from build123d import *

# Parameters (mm, degrees)
CROQUIS1_W              = 3
CROQUIS1_H              = 12.3
SALIENTE_EXTRUIR1_DEPTH = 3


with BuildPart() as part:
    # Croquis1 → Saliente-Extruir1 (new body)
    with BuildSketch(Plane.XY):
        Polygon((307.259692282, 25.949980259), (346.230835452, 48.449980259), (346.230835452, 93.449980259), (307.259692282, 115.949980259), (268.288549111, 93.449980259), (268.288549111, 48.449980259), align=None)
        with Locations((307.259692282, 70.949980259)):
            Rectangle(CROQUIS1_W, CROQUIS1_H, mode=Mode.SUBTRACT)
        with Locations((332.809217745, 70.949980259)):
            Rectangle(CROQUIS1_W, CROQUIS1_H, mode=Mode.SUBTRACT)
        with Locations((281.710166819, 70.949980259)):
            Rectangle(CROQUIS1_W, CROQUIS1_H, mode=Mode.SUBTRACT)
        Polygon((313.95839878, 94.852480259), (324.610511247, 88.702480259), (326.110511247, 91.30055647), (315.45839878, 97.45055647), align=None, mode=Mode.SUBTRACT)
        Polygon((289.908873317, 88.702480259), (288.408873317, 91.30055647), (299.060985783, 97.45055647), (300.560985783, 94.852480259), align=None, mode=Mode.SUBTRACT)
        Polygon((300.560985783, 47.047480259), (289.908873317, 53.197480259), (288.408873317, 50.599404048), (299.060985783, 44.449404048), align=None, mode=Mode.SUBTRACT)
        Polygon((324.610511247, 53.197480259), (326.110511247, 50.599404048), (315.45839878, 44.449404048), (313.95839878, 47.047480259), align=None, mode=Mode.SUBTRACT)
    extrude(amount=SALIENTE_EXTRUIR1_DEPTH)


solid = part.part
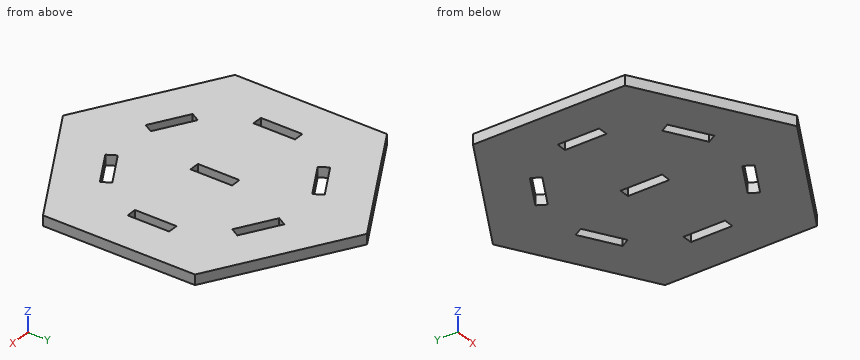
Work out the finished part from the listing and answer in its coordinate system (mm). Round coordinates to 2 decimals unless told otherwise and drop trailing zeros. Order: outer loops, then holes, each group sorted by start corner. A loop starts at its lowest first (then second) coordinate and runs counter-clockwise, first axis right, second up. Notation, with made-up numbers: M 89,71.25 L 147,71.25 A18 cw 147,94.25 Z; hole C 79.25,13 d2. An arc over 180 degrees is marked long. Put each result on its own line as item: value. Start each with the question number.
Q1. Section D-D, the plane y = 104 is taken. Write down the section's boundary in (x, z).
Q2. Section A-A, the plane x = 332.5 is taken. Write down the section's boundary in (y, z), and give its area (3 significant figures).
Q3. Flat-ended cylindrical pins translate along their axes: pin 1 (0.9 mm diameter, centred on x = 332.5, z = 1, fed in from +Y); pin 2 (1.5 mm diameter, centred on x = 282, z = 1, fed in from -Y). Find the tip coordinate at first contact, or state that the pin passes through.
Q4. Straight lines are drawn through the part: L1, parallel to X at y = 65, z = 2; L2, parallel to Y at x = 289.5, z = 1.4; L3, parallel to X at y = 53, z = 0.25. For each, find the intervals that lie inside material, in ascending order. Write a range as [from, to].
Q5. Section C-C, the plane x = 293.5 is taken. Write down the section's boundary in (y, z), and give its area (3 significant figures).
Q6. Section B-B, the plane z = 1.6 is taken. Give the number of separate pieces and of enclosed holes in the cut face, and give its area (3 significant figures).
Findings below:
1. outline: M 286.56,0 L 327.96,0 L 327.96,3 L 286.56,3 Z
2. outline: M 40.52,0 L 64.8,0 L 64.8,3 L 40.52,3 Z; M 77.1,0 L 101.38,0 L 101.38,3 L 77.1,3 Z
2. area: 146 mm^2
3. pin 1: stops at y = 101.64
3. pin 2: stops at y = 40.1
4. L1: x = [268.29, 280.21], [283.21, 305.76], [308.76, 331.31], [334.31, 346.23]
4. L2: y = [36.2, 49.97], [52.49, 89.41], [91.93, 105.7]
4. L3: x = [268.29, 289.79], [290.25, 324.27], [324.72, 346.23]
5. outline: M 33.89,0 L 47.66,0 L 47.66,3 L 33.89,3 Z; M 51.12,0 L 90.78,0 L 90.78,3 L 51.12,3 Z; M 94.24,0 L 108.01,0 L 108.01,3 L 94.24,3 Z
5. area: 202 mm^2
6. separate pieces: 1
6. enclosed holes: 7
6. area: 5,000 mm^2
